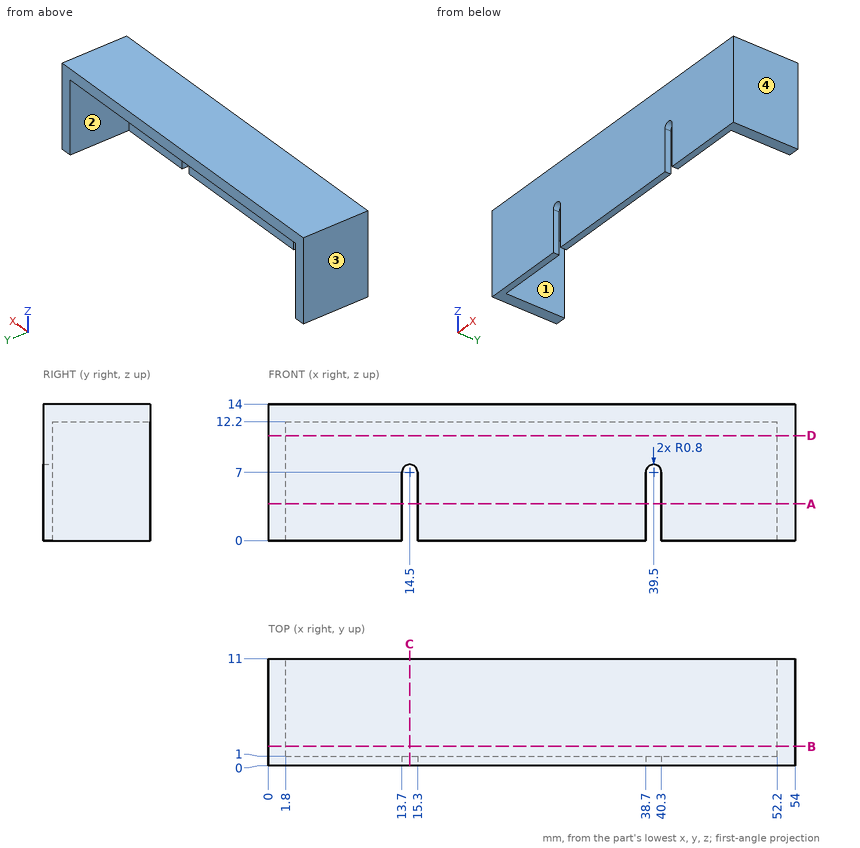
Input: dimensioned drawing with shaded views. Units: mm. Origin: part minimum x, y, z. Coordinates: 2 decimals unless noted, no trailing zeros. Write each loop counter-clockwise with the first axis right and the second up, starting at its lowest first coordinate (ties: lowest second). Pieces come first, ordered by that corner, then holes. Notation, with made-up numbers: (-19, -8) -> (30, -8) arc R19 cw to (30, 29) -> close; hole circle Ø10 at (-2.75, 8). An arc over 180 degrees is marked (long way). Return JSON: item names as keys, results as strings. Group by question number.
1) Ray query, line 1 along X through (y, z) = (5, 4.75); line 2 along Z through (x, y) = (6.5, 3.5); line 3 along Y through (x, z) = (14, 10.75). Return the intervals inside material, ascending.
2) Section query B-B, the plane y = 2. Return loops of the section in (x, z), plus the area to 3 significant figures.
3) Section query A-A, the plane z = 3.75. Return loops of the section in (x, y), plus the area to 3 significant figures.
4) Contact query for a flat-ended pin moving along its axis: P1, Ø3.5, axis at x = 33.5, z = 8.5, coming from the +Y side. Output: stop coordinate, or through.
5) Section query D-D, the plane z = 10.75. Return loops of the section in (x, y), plus the area to 3 significant figures.
6) Mould query, pull axis X, two halves, no side actions, for the marked faces 1, 2, 3 and 4. Classes: +X half, -X half, draft (parallel to the pull), parting line (faces both ways), or undercut.
7) Section query C-C, the plane x = 14.5. Return loops of the section in (y, z), plus the area to 3 significant figures.
From the geometry:
{
 "1": {"line 1": "0 to 1.8, 52.2 to 54", "line 2": "12.2 to 14", "line 3": "0 to 1"},
 "2": {"outline": "(0, 0) -> (1.8, 0) -> (1.8, 12.2) -> (52.2, 12.2) -> (52.2, 0) -> (54, 0) -> (54, 14) -> (0, 14) -> close", "area": "141 mm²"},
 "3": {"outline": "(0, 0) -> (13.7, 0) -> (13.7, 1) -> (1.8, 1) -> (1.8, 11) -> (0, 11) -> close; (15.3, 0) -> (38.7, 0) -> (38.7, 1) -> (15.3, 1) -> close; (40.3, 0) -> (54, 0) -> (54, 11) -> (52.2, 11) -> (52.2, 1) -> (40.3, 1) -> close", "area": "86.8 mm²"},
 "4": {"P1": "y = 1"},
 "5": {"outline": "(0, 0) -> (54, 0) -> (54, 11) -> (52.2, 11) -> (52.2, 1) -> (1.8, 1) -> (1.8, 11) -> (0, 11) -> close", "area": "90.0 mm²"},
 "6": {"face 1": "undercut", "face 2": "undercut", "face 3": "-X half", "face 4": "+X half"},
 "7": {"outline": "(0, 7.8) -> (1, 7.8) -> (1, 12.2) -> (11, 12.2) -> (11, 14) -> (0, 14) -> close", "area": "24.2 mm²"}
}
